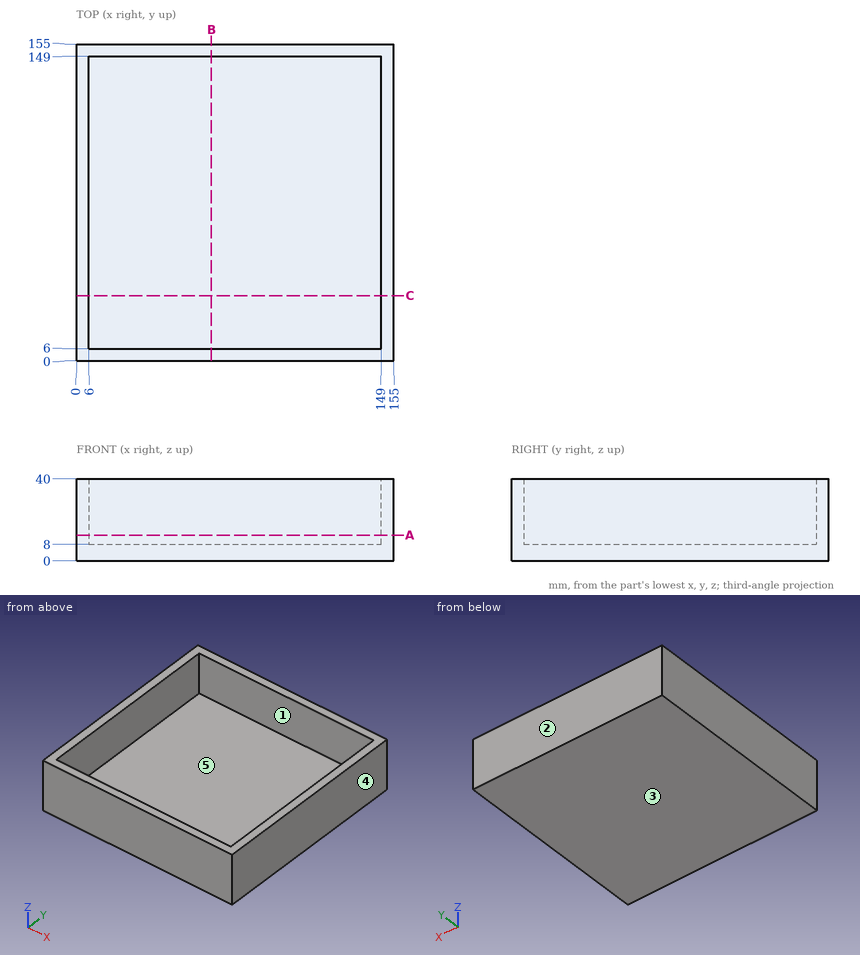
Part print with two shaded views. Sizes in mm from the minimum x, y, z corner. A direction names the side the tool comes from. Coordinates: 2 decimals unless noted, no trailing zeros. Loops run counter-clockwise (first coordinate to the right, second up) from the corner with the lowest first, then second, coordinate; pieces in that order, holes last. Notation, with made-up numbers: (14, -12.5) -> (39, -12.5) arc R6 cw to (39, -2.5) -> close; hole circle Ø4 at (1, 43). An arc over 180 degrees is marked (long way). Answer as a JSON object with one key per item and string values.
Q1. Cut at A-A (z = 12.5). List the corners of the cut face in (x, y), and give its area (3 significant figures).
Report:
{"outline": "(0, 0) -> (155, 0) -> (155, 155) -> (0, 155) -> close; hole (6, 6) -> (149, 6) -> (149, 149) -> (6, 149) -> close", "area": "3,580 mm2"}
Q2. Pull direction X, two halves, no side cores. Call the marked faces 3, 4 and 5: released by +X, released by -X, zero draft, split by the parting line, or undercut.
Report:
{"face 3": "zero draft", "face 4": "released by +X", "face 5": "undercut"}
Q3. Flat gauge pin, fed straight in: P1, Ø1, axis at x = 138, y = 93, coming from the +Z side. Where does the tip first touch, or does it go through?
Report:
{"P1": "stops at z = 8"}
Q4. 3-axis set-ups, long thin cutter, end or side, ignore diameter. For the marked faces 1 and 2: which of +Z, -Z, +X, -X, +Y, -Y reach the whole face in a straight line?
Report:
{"face 1": "+Z", "face 2": "+Z, -Z, +X, -X, +Y"}
Q5. Probe probe 1 along Y at (x, z) = (104, 10); probe 2 along Z at (x, y) = (45, 120). List the from-to ranges inside material, lowest first.
Report:
{"probe 1": "y = 0 to 6, 149 to 155", "probe 2": "z = 0 to 8"}
Q6. Cut at B-B (x = 66). List the corners of the cut face in (y, z).
Report:
{"outline": "(0, 0) -> (155, 0) -> (155, 40) -> (149, 40) -> (149, 8) -> (6, 8) -> (6, 40) -> (0, 40) -> close"}
